Could you check a few things on this model? Use its own coordinates, in mm. A direction names the side the tool comes from. Give positions to 0.01 mm unless a question says otherwise; leave off trailing zeros. Order: outer loops, then holes, each group sorted by start corner. A loop starts at its lowest first (then second) coordinate and runs counter-clockwise, first axis right, second up. Notation, with made-up numbers: M 7,15.25 L 29,15.25 A35 cw 29,47.25 Z; hole C 49,-28 d3. An arc over 180 degrees is marked long. Return JSON: item names as keys, results as strings. Group by question number.
```python
from build123d import *

# Parameters (mm, degrees)
SKETCH_1_W          = 37
SKETCH_1_H          = 19.73
EXTRUDE_1_DEPTH     = 12
SKETCH_2_R          = 1.5
CUT_EXTRUDE_1_DEPTH = 25.157156807
FILLET_2_R          = 4
SKETCH_3_R          = 2.5
CUT_EXTRUDE_2_DEPTH = 30
SKETCH_4_W          = 5
SKETCH_4_H          = 3
EXTRUDE_2_DEPTH     = 4.7
SKETCH_5_R          = 1.5
CUT_EXTRUDE_3_DEPTH = 27.302247528
FILLET_3_R          = 1


with BuildPart() as part:
    # 草图1 → 凸台-拉伸1 (new body)
    with BuildSketch(Plane(origin=(0, 0, 0), x_dir=(1, 0, 0), z_dir=(0, 1, 0))):
        Rectangle(SKETCH_1_W, SKETCH_1_H)
    extrude(amount=EXTRUDE_1_DEPTH)

    # 草图2 → 切除-拉伸1 (cut, through all)
    with BuildSketch(Plane(origin=(0, 12, 0), x_dir=(1, 0, 0), z_dir=(0, 1, 0))):
        with Locations((-18.5, 0)):
            Circle(SKETCH_2_R)
    extrude(amount=-CUT_EXTRUDE_1_DEPTH, mode=Mode.SUBTRACT)

    # 圆角2
    fillet_2_edges = [part.edges().sort_by_distance(p)[0] for p in [
        (0, 12, -9.865),
        (0, 0, -9.865),
        (0, 0, 9.865),
        (0, 12, 9.865),
    ]]
    fillet(fillet_2_edges, radius=FILLET_2_R)

    # 草图3 → 切除-拉伸2 (cut)
    with BuildSketch(Plane.ZY.offset(18.5)):
        with Locations((-4.035, 6)):
            Circle(SKETCH_3_R)
    extrude(amount=-CUT_EXTRUDE_2_DEPTH, mode=Mode.SUBTRACT)

    # 草图4 → 凸台-拉伸2 (add)
    with BuildSketch(Plane(origin=(18.5, 0, 0), x_dir=(0, 0, -1), z_dir=(1, 0, 0))):
        with Locations((4.035, 6)):
            Rectangle(SKETCH_4_W, SKETCH_4_H)
    extrude(amount=EXTRUDE_2_DEPTH)

    # 草图5 → 切除-拉伸3 (cut, through all)
    with BuildSketch(Plane(origin=(0, 7.5, 0), x_dir=(1, 0, 0), z_dir=(0, 1, 0))):
        with Locations(Location((20.7, 4.035, 0), (0, 0, 270))):
            Circle(SKETCH_5_R)
    extrude(amount=-CUT_EXTRUDE_3_DEPTH, mode=Mode.SUBTRACT)

    # 圆角3
    fillet_3_edges = [part.edges().sort_by_distance(p)[0] for p in [
        (23.2, 6, -6.535),
        (23.2, 6, -1.535),
    ]]
    fillet(fillet_3_edges, radius=FILLET_3_R)


solid = part.part
```
1. I need wall thicknesses on L1, parallel to X at y = 2.75, z = -7; L2, parallel to Y at x = 9, z = -3; L3, parallel to Y at x = 9.5, z = -2. Which ranges of each line are inside material? Lowest first, please. Write a range as from..to.
2. Which directions (+Z, -Z, +X, -X, +Y, -Y) give clear straight access to the entire face, cutting with the end or side of a thin tool? Please do faces 4 (the flat face through (22, 4.5, -3)), 5 (the flat face through (20, 6, -6.535)), 6 (the cylindrical face through (-3.71, 8.48, -4.36)), 7 (the flat face through (22, 7.5, -3)), 8 (the flat face through (-18.5, 6, 6)).
3. Imagine slicing it at C-C, the plane y = 6. Please give me the cut outline in (x, z) (3 decimals).
4. Imagine slicing it at A-A, the plane x = 20.7. Please give me the cut outline in (y, z) (3 decimals), plus the area to 3 significant figures.
5. If we mould it in two halves opening along Y, with no side actions, what happens to faces 1 (the flat face through (0, 6, 9.865)), 2 (the cylindrical face through (0.26, 10.8, 8.72)), 3 (the flat face through (11.5, 6, -4))? For each: pulls with the +Y half, pulls with the -Y half, needs draft (parallel to the pull), parting line crosses it, or undercut.
6. Imagine slicing it at B-B, the plane x = 5.5. Please give me the cut outline in (y, z) (3 decimals).
7. For pin 1 (0.9 mm diameter, centred on x = 21, y = 6, fed in from +Z) (3 decimals); pin 2 (4 mm diameter, centred on y = 10, z = -7.5, fed in from +X); pin 3 (3.5 mm diameter, centred on x = 20.7, z = -4.035, fed in from -Y), each with a flat end and sliding along its axis, tell me the tip position at first contact or that it passes through.
8. Imagine slicing it at D-D, the plane z = -3. Please give me the cut outline in (x, y).
Values:
{
 "1": {"L1": "x = -18.5..18.5", "L2": "y = 0..3.72, 8.28..12", "L3": "y = 0..4.55, 7.45..12"},
 "2": {"face 4": "+Z, -Z, +X, -Y", "face 5": "-Z, +X, +Y, -Y", "face 6": "-X", "face 7": "+Z, -Z, +X, +Y", "face 8": "+Z, -Z, -X, +Y, -Y"},
 "3": {"outline": "M -18.5,-9.865 L 18.5,-9.865 L 18.5,-6.535 L 22.2,-6.535 A1 ccw 23.2,-5.535 L 23.2,-2.535 A1 ccw 22.2,-1.535 L 18.5,-1.535 L 18.5,9.865 L -18.5,9.865 L -18.5,1.5 A1.5 cw -18.5,-1.5 L -18.5,-1.535 L 11.5,-1.535 L 11.5,-6.535 L -18.5,-6.535 Z; hole C 20.7,-4.035 d3"},
 "4": {"outline": "M 4.5,-6.535 L 7.5,-6.535 L 7.5,-5.535 L 4.5,-5.535 Z; M 4.5,-2.535 L 7.5,-2.535 L 7.5,-1.535 L 4.5,-1.535 Z", "area": "6.00 mm²"},
 "5": {"face 1": "needs draft", "face 2": "pulls with the +Y half", "face 3": "undercut"},
 "6": {"outline": "M 0,-5.865 A4 ccw 4,-9.865 L 8,-9.865 A4 ccw 12,-5.865 L 12,5.865 A4 ccw 8,9.865 L 4,9.865 A4 ccw 0,5.865 Z; hole C 6,-4.035 d5"},
 "7": {"pin 1": "stops at z = -1.535", "pin 2": "stops at x = 18.5", "pin 3": "stops at y = 4.5"},
 "8": {"outline": "M -18.5,0 L 18.5,0 L 18.5,4.5 L 19.61,4.5 L 19.61,7.5 L 18.5,7.5 L 18.5,12 L -18.5,12 L -18.5,8.28 L 11.5,8.28 L 11.5,3.72 L -18.5,3.72 Z; M 21.79,4.5 L 23.2,4.5 L 23.2,7.5 L 21.79,7.5 Z"}
}
